CAD build for the part. Positions are in the model's coordinates, mm. Round coordinates to 2 decimals unless told otherwise and drop trailing zeros. Order: outer loops, then holes, each group sorted by start corner. A loop starts at its lowest first (then second) coordinate and runs counter-clockwise, first axis right, second up. Notation, with made-up numbers: M 0,35.25 L 28,35.25 A8 ccw 28,41.25 Z; hole C 86.25,26.25 d8. An arc over 180 degrees is marked long. Put each result on its own line as item: value.
```python
from build123d import *

# Parameters (mm, degrees)
BASE_FLANGE1_DEPTH = 1
SKETCH2_R          = 2.5
CUT_EXTRUDE1_DEPTH = 10
FILLET1_R          = 3


# Sheet-metal steps are written as plain solids
with BuildPart() as part:
    # Sketch1 → Base-Flange1 (new body)
    with BuildSketch(Plane.XY):
        Polygon((104, 853), (16, 853), (16, 107.151941455), (170, 18.24), (170, 123.634882233), (104, 161.74), align=None)
    extrude(amount=-BASE_FLANGE1_DEPTH)

    # Sketch2 → Cut-Extrude1 (cut)
    with BuildSketch(Plane(origin=(0, 0, -1), x_dir=(-1, 0, 0), z_dir=(0, 0, -1))):
        with Locations((-22, 824)):
            Circle(SKETCH2_R)
        with Locations((-98, 824)):
            Circle(SKETCH2_R)
        with Locations((-98, 656)):
            Circle(SKETCH2_R)
        with Locations((-98, 488)):
            Circle(SKETCH2_R)
        with Locations((-98, 320)):
            Circle(SKETCH2_R)
        with Locations((-22, 656)):
            Circle(SKETCH2_R)
        with Locations((-22, 488)):
            Circle(SKETCH2_R)
        with Locations((-22, 320)):
            Circle(SKETCH2_R)
        with Locations((-22, 152)):
            Circle(SKETCH2_R)
        with Locations((-98, 177)):
            Circle(SKETCH2_R)
        with Locations((-140, 134.564882233)):
            Circle(SKETCH2_R)
        with Locations((-130, 50.734882233)):
            Circle(SKETCH2_R)
        with Locations((-43.397459622, 100.734882233)):
            Circle(SKETCH2_R)
    extrude(amount=-CUT_EXTRUDE1_DEPTH, mode=Mode.SUBTRACT)

    # Fillet1
    fillet1_edges = [part.edges().sort_by_distance(p)[0] for p in [
        (104, 161.74, -0.5),
        (170, 123.634882233, -0.5),
        (170, 18.24, -0.5),
        (16, 107.151941455, -0.5),
        (16, 853, -0.5),
        (104, 853, -0.5),
    ]]
    fillet(fillet1_edges, radius=FILLET1_R)


solid = part.part
```
Item 1: Band-saw the part on B-B on z = -0.45. State how many separate pieces and enclosed holes the cut face has, and give its area (3 significant figures).
Answers below:
separate pieces: 1
enclosed holes: 13
area: 74,600 mm²
Item 2: Band-saw the part on A-A on y = 761.5. Give the cut face in (x, z).
Answers below:
outline: M 16,-1 L 104,-1 L 104,0 L 16,0 Z
Item 3: Probe line 1 along X through (y, z) = (656, -0.3); line 2 along Y through (x, z) = (98, -0.35); line 3 along X through (y, z) = (319, -0.5). List the from-to ranges inside material, lowest first. Write a range as [from, to].
Answers below:
line 1: [16, 19.5], [24.5, 95.5], [100.5, 104]
line 2: [59.81, 174.5], [179.5, 317.5], [322.5, 485.5], [490.5, 653.5], [658.5, 821.5], [826.5, 853]
line 3: [16, 19.71], [24.29, 95.71], [100.29, 104]
Item 4: Mould opens along Y. For faces 1 (the flat face through (90.464, 64.16, -0.493)), 2 (the flat face through (137.441, 142.433, -0.493)), 3 (the flat face through (58, 443, 0)) say: pulls with the +Y half, pulls with the -Y half, needs draft (parallel to the pull), parting line crosses it, or undercut.
Answers below:
face 1: pulls with the -Y half
face 2: pulls with the +Y half
face 3: needs draft
Item 5: Band-saw the part on C-C on y = 72. Give the cut face in (x, z).
Answers below:
outline: M 76.88,-1 L 170,-1 L 170,0 L 76.88,0 Z
